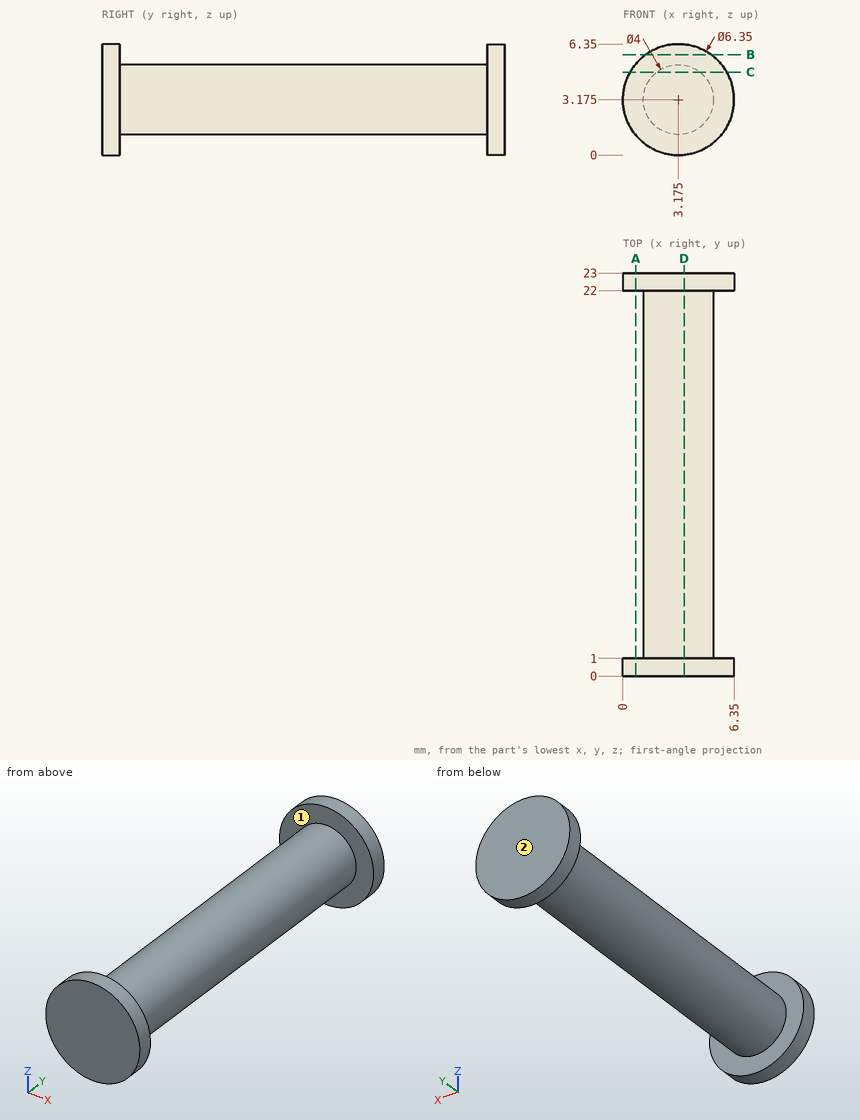
Geometry: see drawing. Coordinates: mm, zero at the bounding-box minimum. A direction names the side the tool comes from. Give positions to 0.01 mm unless a question says otherwise; leave off trailing zeros. Order: outer loops, then holes, each group sorted by start corner. A loop starts at its lowest first (then second) coordinate and runs counter-clockwise, first axis right, second up. Notation, with made-up numbers: M -27,48 L -2,48 A14 cw -2,61 Z; hole C -25,7.5 d9. An arc over 180 degrees is marked long. Answer as CSV lines item,"result". Start each with the question number.
1) Cut plane D-D (x = 3.5). Output: boundary loops of the cut face in (y, z).
2) Line query: line 1 (Y direction, x = 1.75, z = 5); line 2 (X direction, y = 17.5, z = 3.25); line 3 (X direction, y = 3, z = 4.5). Output: solid intervals per line, ascending. Write a range as from..to.
3) Cut plane C-C (z = 4.75). Output: boundary loops of the cut face in (x, y), then the cut area to 3 significant figures.
4) First-contact query: P1, Ø1.5, axis at y = 16.5, z = 3.5, coming from the -X side (3 decimals). Flat tip, straight axial feed; report the tip coordinate or a pass-through.
5) Cut plane A-A (x = 0.75). Output: boundary loops of the cut face in (y, z), then the cut area to 3 significant figures.
6) Cut plane B-B (z = 5.75). Output: boundary loops of the cut face in (x, y), then the cut area to 3 significant figures.
7) Set-up query: the marked faces 1 and 2. Return all of +Z, -Z, +X, -X, +Y, -Y with unobstructed straight access to the full face (end or side cutting, diameter ignored); none if empty.
Findings below:
1,outline,"M 0,0.02 L 1,0.02 L 1,1.2 L 22,1.2 L 22,0.02 L 23,0.02 L 23,6.33 L 22,6.33 L 22,5.15 L 1,5.15 L 1,6.33 L 0,6.33 Z"
2,line 1,"y = 0..1, 22..23"
2,line 2,"x = 1.18..5.17"
2,line 3,"x = 1.68..4.67"
3,outline,"M 0.42,0 L 5.93,0 L 5.93,1 L 4.41,1 L 4.41,22 L 5.93,22 L 5.93,23 L 0.42,23 L 0.42,22 L 1.94,22 L 1.94,1 L 0.42,1 Z"
3,area,"62.8 mm²"
4,P1,"stops at x = 1.175"
5,outline,"M 0,1.13 L 1,1.13 L 1,5.22 L 0,5.22 Z; M 22,1.13 L 23,1.13 L 23,5.22 L 22,5.22 Z"
5,area,"8.20 mm²"
6,outline,"M 1.32,0 L 5.03,0 L 5.03,1 L 1.32,1 Z; M 1.32,22 L 5.03,22 L 5.03,23 L 1.32,23 Z"
6,area,"7.43 mm²"
7,face 1,"none"
7,face 2,"+Z, -Z, +X, -X, +Y"
